Read the model definition and answer for the solid it produces. Units are mm, in the model's axes. Face numbers are marked on the shaded views. A direction names the side the tool comes from. Coordinates: 2 decimals unless noted, no trailing zeros. Loops run counter-clockwise (first coordinate to the right, second up) from the corner with the lowest first, then second, coordinate; pieces in that order, holes last.
Autodesk Fusion 360 part; units mm, degrees
sketch "Sketch1" plane through (0, 0, 0) normal (0, 0, 1) x (1, 0, 0)
  line L0 (0, 0) -> (3, 0)
  line L1 (3, 0) -> (3, 80)
  line L2 (3, 80) -> (0, 80)
  line L3 (0, 77) -> (0, 0)
  line L4 (0, 80) -> (-57, 80)
  line L5 (-57, 80) -> (-57, 77)
  line L6 (-54, 77) -> (0, 77)
  line L7 (-54, 77) -> (-54, 65)
  line L8 (-54, 65) -> (-57, 65)
  line L9 (-57, 65) -> (-57, 77)
  dimension "d1" = 80
  dimension "d2" = 3
  dimension "d3" = 60
  dimension "d4" = 3
  dimension "d5" = 15
  dimension "d6" = 3
extrude "Extrude1" add sketch "Sketch1" along normal blind 8
fillet "Fillet1" radius 1 8 edges at (0, 77, 4) (-54, 77, 4) (-54, 65, 4) (-57, 65, 4) (-57, 80, 4) (3, 80, 4) (3, 0, 4) (0, 0, 4)
sketch "Sketch2" plane through (3, 0, 0) normal (1, 0, 0) x (0, 1, 0)
  line L0 (1, 8) -> (1, 0)
  line L1 (1, 0) -> (79, 0)
  line L2 (79, 0) -> (79, 8)
  line L3 (79, 8) -> (1, 8)
  line L4 (80, 0) -> (80, 8)
  point P0 (61.5, 3.944)
  point P1 (18.5, 3.944)
  dimension "d11" = 43
  dimension "d12" = 18.5
hole "Hole1" at (3, 61.5, 3.944) at (3, 18.5, 3.944) direction (-1, 0, 0) diameter 5 depth 3 tip angle 118
equation "d12 = ( ( 80 - 43 ) / 2 ) * 1 mm"
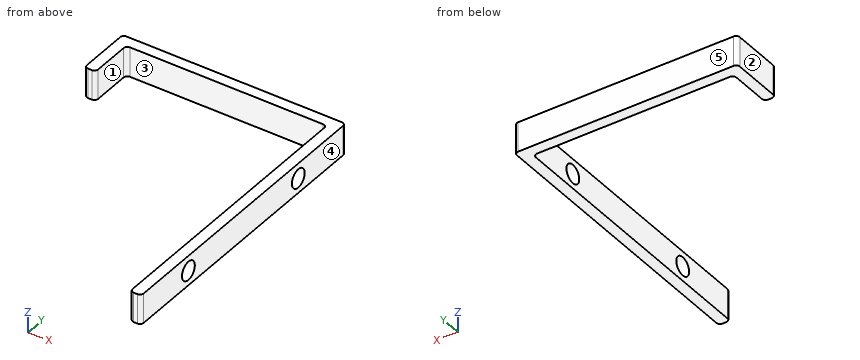
Item 1: Find the intervals of material crossed by line 1 along Z through (x, y) = (2.05, 61.5); line 2 along X through (y, z) = (68.5, 2.5); line 3 along Y through (x, z) = (-31, 1.75), in increasing order.
Numbers:
line 1: z = 0 to 1.44, 6.44 to 8
line 2: x = -57 to -54, 0 to 3
line 3: y = 77 to 80
Item 2: A cutting plane is placed at D-D on y = 41.5. Determine the outline of the cut face in (x, z), then the cut area to 3 significant figures.
Numbers:
outline: (0, 0) - (3, 0) - (3, 8) - (0, 8) - close
area: 24.0 mm2
Item 3: Which of the six approach directions +Z, -Z, +X, -X, +Y, -Y give full straight-line access (tool end or side, diameter ignored) to the marked faces 1 and 2?
Numbers:
face 1: +Z, -Z, -Y
face 2: +Z, -Z, -X, +Y, -Y
Item 4: Determine the mould class of the marked faces 3, 4 and 5 for opening direction X: released by +X, released by -X, zero draft, split by the parting line, or undercut.
Numbers:
face 3: undercut
face 4: released by +X
face 5: zero draft
Item 5: A cutting plane is placed at B-B on z = 2.25. Determine the outline of the cut face in (x, y), then the cut area to 3 significant figures.
Numbers:
outline: (-57, 66) arc R1 ccw to (-56, 65) - (-55, 65) arc R1 ccw to (-54, 66) - (-54, 76) arc R1 cw to (-53, 77) - (-1, 77) arc R1 cw to (0, 76) - (0, 63.34) - (3, 63.34) - (3, 79) arc R1 ccw to (2, 80) - (-56, 80) arc R1 ccw to (-57, 79) - close; (0, 1) arc R1 ccw to (1, 0) - (2, 0) arc R1 ccw to (3, 1) - (3, 16.66) - (0, 16.66) - close; (0, 20.34) - (3, 20.34) - (3, 59.66) - (0, 59.66) - close
area: 424 mm2
Item 6: A cutting plane is placed at A-A on y = 18.5. Determine the outline of the cut face in (x, z), then the cut area to 3 significant figures.
Numbers:
outline: (0, 0) - (3, 0) - (3, 1.44) - (0, 1.44) - close; (0, 6.44) - (3, 6.44) - (3, 8) - (0, 8) - close
area: 9.00 mm2
Item 7: Given pin 1 (0.5 mm diameter, centred on x = -55.5, z = 5.5, fed in from -Y); pin 2 (2.5 mm diameter, centred on y = 21, z = 5, fed in from -X); pin 3 (3 mm diameter, centred on x = -39.5, z = 2.5, fed in from -Y), each flat-ended and moving along its own axis, determine where each tip first touches the part or whether it passes through.
Numbers:
pin 1: stops at y = 65
pin 2: stops at x = 0
pin 3: stops at y = 77
Item 8: A cutting plane is placed at C-C on x = -29. Determine the outline of the cut face in (y, z).
Numbers:
outline: (77, 0) - (80, 0) - (80, 8) - (77, 8) - close
